Build history of the part. All positions in model axes, mm. Give positions to 0.01 mm unless a question says otherwise; leave off trailing zeros. Order: outer loops, then holes, each group sorted by start corner. A loop starts at its lowest first (then second) coordinate and runs counter-clockwise, first axis right, second up. Notation, with made-up numbers: (36.5, 70.5) - (91.5, 70.5) arc R25 ccw to (91.5, 102.5) - close; hole circle Ø7 at (-39.5, -32). An arc over 180 degrees is marked (long way). Use a Markdown table: item, result. Add a question column.
(1) Slice it at D-D (y = -24). Write the cut outline in (x, z), then the cut area to 3 significant figures.
(2) Slice it at B-B (x = 1.85). Write the cut outline in (y, z).
(3) Flat gauge pins, fed straight in: pin 1 (0.9 mm diameter, centred on x = 4, y = -44, fed in from -Z); pin 2 (1.5 mm diameter, centred on y = -9.5, z = 59.5, fed in from -X); pin 3 (1.5 mm diameter, centred on x = 5, z = 62, fed in from -Y); pin 4 (1.5 mm diameter, centred on x = 4, y = -44.5, fed in from +Z). Where does each tip first touch, or does it go through?
(4) Slice it at A-A (y = -34). Write the cut outline in (x, z).
(5) Wall check: line 1 (Z direction, x = 2.25, y = -27); line 2 (Y direction, x = 1.05, z = 57.5); line 3 (Z direction, x = 4.4, y = -45). Give the ranges that are in metal, low to high.
(6) Slice it at C-C (z = 60). Write the cut outline in (x, y), then the cut area to 3 significant figures.
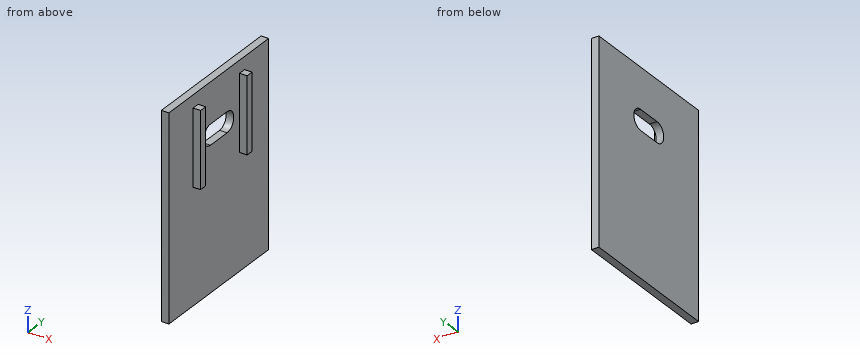
from build123d import *

# Parameters (mm, degrees)
F0_W     = 60
F0_H     = 80
F1_DEPTH = 3
F2_W     = 3
F2_H     = 30
F3_DEPTH = 3


with BuildPart() as f1:
    # F0 (on Right) → F1 (new body)
    with BuildSketch(Plane.YZ):
        with Locations((-30, 40)):
            Rectangle(F0_W, F0_H)
        with BuildLine():
            ThreePointArc((-35, 56), (-39, 60), (-35, 64))
            Line((-35, 64), (-25, 64))
            ThreePointArc((-25, 64), (-21, 60), (-25, 56))
            Line((-25, 56), (-35, 56))
        make_face(mode=Mode.SUBTRACT)
    extrude(amount=F1_DEPTH)

    # F2 (on face) → F3 (join)
    with BuildSketch(Plane.YZ.offset(3)):
        with Locations((-44, 60)):
            Rectangle(F2_W, F2_H)
        with Locations((-16, 60)):
            Rectangle(F2_W, F2_H)
    extrude(amount=F3_DEPTH)


solid = f1.part
Solution:
| question | item | result |
|---|---|---|
| 1 | outline | (0, 0) - (3, 0) - (3, 56.13) - (0, 56.13) - close; (0, 63.87) - (3, 63.87) - (3, 80) - (0, 80) - close |
| 1 | area | 217 mm2 |
| 2 | outline | (-60, 0) - (0, 0) - (0, 80) - (-60, 80) - close; hole (-35, 56) - (-25, 56) arc R4 ccw to (-25, 64) - (-35, 64) arc R4 ccw to start |
| 3 | pin 1 | z = 45 |
| 3 | pin 2 | x = 0 |
| 3 | pin 3 | y = -45.5 |
| 3 | pin 4 | z = 75 |
| 4 | outline | (0, 0) - (3, 0) - (3, 56) - (0, 56) - close; (0, 64) - (3, 64) - (3, 80) - (0, 80) - close |
| 5 | line 1 | 0 to 56, 64 to 80 |
| 5 | line 2 | -60 to -38.12, -21.88 to 0 |
| 5 | line 3 | 45 to 75 |
| 6 | outline | (0, -60) - (3, -60) - (3, -45.5) - (6, -45.5) - (6, -42.5) - (3, -42.5) - (3, -39) - (0, -39) - close; (0, -21) - (3, -21) - (3, -17.5) - (6, -17.5) - (6, -14.5) - (3, -14.5) - (3, 0) - (0, 0) - close |
| 6 | area | 144 mm2 |
